```python
from build123d import *

# Parameters (mm, degrees)
SKETCH_1_W          = 68
SKETCH_1_H          = 80
EXTRUDE_1_DEPTH     = 3
SKETCH_2_R          = 1.575
CUT_EXTRUDE_1_DEPTH = 53.583267301
SKETCH_4_W          = 68
SKETCH_4_H          = 16.52
CUT_EXTRUDE_2_DEPTH = 53.583267301
SKETCH_5_W          = 68
SKETCH_5_H          = 3
EXTRUDE_2_DEPTH     = 11.8
FILLET_1_R          = 3
SKETCH_6_R          = 2
CUT_EXTRUDE_3_DEPTH = 14.5
FILLET_2_R          = 35


with BuildPart() as part:
    # 草图1 → 凸台-拉伸1 (new body)
    with BuildSketch(Plane.XY):
        Rectangle(SKETCH_1_W, SKETCH_1_H)
    extrude(amount=EXTRUDE_1_DEPTH)

    # 草图2 → 切除-拉伸1 (cut, through all)
    with BuildSketch(Plane.XY.offset(3)):
        with Locations((-19.516147161, 24.516147161)):
            Circle(SKETCH_2_R)
        with Locations((19.516147161, 24.516147161)):
            Circle(SKETCH_2_R)
        with Locations((-19.516147161, -14.516147161)):
            Circle(SKETCH_2_R)
        with Locations((19.516147161, -14.516147161)):
            Circle(SKETCH_2_R)
    extrude(amount=-CUT_EXTRUDE_1_DEPTH, mode=Mode.SUBTRACT)

    # 草图4 → 切除-拉伸2 (cut, through all)
    with BuildSketch(Plane.XY.offset(3)):
        with Locations((0, -31.74)):
            Rectangle(SKETCH_4_W, SKETCH_4_H)
    extrude(amount=-CUT_EXTRUDE_2_DEPTH, mode=Mode.SUBTRACT)

    # 草图5 → 凸台-拉伸2 (add)
    with BuildSketch(Plane.XY.offset(3)):
        with Locations((0, -21.98)):
            Rectangle(SKETCH_5_W, SKETCH_5_H)
    extrude(amount=EXTRUDE_2_DEPTH)

    # 圆角1
    fillet_1_edges = [part.edges().sort_by_distance(p)[0] for p in [
        (0, -23.48, 0),
        (0, -20.48, 3),
    ]]
    fillet(fillet_1_edges, radius=FILLET_1_R)

    # 草图6 → 切除-拉伸3 (cut)
    with BuildSketch(Plane(origin=(0, -20.48, 0), x_dir=(1, 0, 0), z_dir=(0, 1, 0))):
        with Locations(Location((24, -9.8, 0), (0, 0, 270))):
            Circle(SKETCH_6_R)
        with Locations(Location((-24, -9.8, 0), (0, 0, 270))):
            Circle(SKETCH_6_R)
    extrude(amount=-CUT_EXTRUDE_3_DEPTH, mode=Mode.SUBTRACT)

    # 圆角2
    # the kernel refuses this fillet: 35 mm, written as the material it takes off along each edge
    with BuildSketch(Plane(origin=(34, 40, -87.5), x_dir=(-1, 0, 0), z_dir=(0, 0, 1)), Plane(origin=(-34, 40, -87.5), x_dir=(0, -1, 0), z_dir=(0, 0, 1))) as fillet_2_piece_1:
        with BuildLine():
            CenterArc((FILLET_2_R, FILLET_2_R), FILLET_2_R, 180, 90)
            Line((0, FILLET_2_R), (0, 0))
            Line((0, 0), (FILLET_2_R, 0))
        make_face()
    extrude(amount=178, mode=Mode.SUBTRACT)


solid = part.part
```
Work out the finished part from the listing and answer in its coordinate system (mm). A direction names the side the tool comes from. Give positions to 0.01 mm unless a question says otherwise; leave off trailing zeros. Loops run counter-clockwise (first coordinate to the right, second up) from the corner with the lowest first, then second, coordinate; pieces in that order, holes last. Notation, with made-up numbers: (39, 82.5) -> (52, 82.5) arc R12 cw to (52, 105.5) -> close; hole circle Ø8 at (36, 89). An arc over 180 degrees is marked (long way). Write item = value, one per line. Start each with the question number.
(1) Find section A-A on z = 9.8. Give the vertices of the cut face in (x, y).
(2) Find section B-B on x = 24. Give the vertices of the cut face in (y, z).
(3) Given pin 1 Ø17 at (x, y) = (14.5, -3) entering from +Z; pin 2 Ø4.5 at (x, z) = (24, 9.8) entering from +Y, each flat-ended and moving along its own axis, determine where each tip first touches the part or whether it passes through.
(4) Find section C-C on x = 5.5. Give the vertices of the cut face in (y, z).
(5) Find section D-D on y = 3. Give the vertices of the cut face in (x, z).
(6) Find the intervals of material crossed by probe 1 along X at (y, z) = (-21.65, 9.8); probe 2 along X at (y, z) = (24.5, 2.25); probe 3 along Y at (x, z) = (18.5, 2), in increasing order. Write a range as from..to.
(7) The mould has two halves that part along X. Classify faces 3 (the cylindrical face through (0.48, -19.58, 3.86)), 4 (the flat face through (-34, -12, 2)), 5 (the cylindrical face through (17.943, -14.447, 1.521)): +X half, -X half, draft (parallel to the pull), parting line (faces both ways), or undercut.
(8) Which of the six approach directions +Z, -Z, +X, -X, +Y, -Y give full straight-line access (tool end or side, diameter ignored) to faces 1 (the cylindrical face through (0.48, -22.62, 0.9)), 2 (the flat face through (0, -20.48, 10))?
From the geometry:
q1.outline = (-34, -23.48) -> (-26, -23.48) -> (-26, -20.48) -> (-34, -20.48) -> close; (-22, -23.48) -> (22, -23.48) -> (22, -20.48) -> (-22, -20.48) -> close; (26, -23.48) -> (34, -23.48) -> (34, -20.48) -> (26, -20.48) -> close
q2.outline = (-23.48, 3) arc R3 ccw to (-20.48, 0) -> (29.49, 0) -> (29.49, 3) -> (-17.48, 3) arc R3 cw to (-20.48, 6) -> (-20.48, 7.8) -> (-23.48, 7.8) -> close; (-23.48, 11.8) -> (-20.48, 11.8) -> (-20.48, 14.8) -> (-23.48, 14.8) -> close
q3.pin_1 = 3
q3.pin_2 = -20.48
q4.outline = (-23.48, 3) arc R3 ccw to (-20.48, 0) -> (39.39, 0) -> (39.39, 3) -> (-17.48, 3) arc R3 cw to (-20.48, 6) -> (-20.48, 14.8) -> (-23.48, 14.8) -> close
q5.outline = (-34, 0) -> (34, 0) -> (34, 3) -> (-34, 3) -> close
q6.probe_1 = -34..-26, -22..22, 26..34
q6.probe_2 = -28.06..-21.09, -17.94..17.94, 21.09..28.06
q6.probe_3 = -23.31..-15.72, -13.31..23.31, 25.72..34.06
q7.face_3 = draft
q7.face_4 = -X half
q7.face_5 = undercut
q8.face_1 = -Z, +X, -X, -Y
q8.face_2 = +Z, +X, -X, +Y
